Build history of the part. All positions in model axes, mm. A direction names the side the tool comes from. Coordinates: 2 decimals unless noted, no trailing zeros. Loops run counter-clockwise (first coordinate to the right, second up) from the corner with the lowest first, then second, coordinate; pieces in that order, holes last.
(1) Tool access for faces 1 (the face through (-83.577, 56.38, -1.565)), 2 (the face through (-75, 46, -91.148)), 3 (the face through (-78.03, 49.35, -92.71)), 4 (the face through (-66.658, 34.949, -1.565)), 5 (the face through (-75, 46, -3.175)): list every direction of +Z, -Z, +X, -X, +Y, -Y with a clear straight run to the whole face (end or side of a thin tool).
(2) Wall check: L1, parallel to Z at x = -86.5, y = 60 (3 decimals); L2, parallel to X at y = 50, z = -16; L3, parallel to X at y = 59.5, z = -41. Give the ranges that are in metal, low to high.
(3) Slice it at A-A (x = -67). Give the cut face in (y, z) (3 decimals), and give its area (3 significant figures).
(4) Slice it at B-B (z = -26.5). Give the cut face in (x, y), and give its area (3 significant figures).
(5) Slice it at C-C (y = 27). Give the cut face in (x, z) (3 decimals).
(6) Flat gauge pins, fed straight in: P1, Ø11.5, axis at x = -61.5, y = 28.5, coming from the -Z side; P2, Ø2, axis at y = 53, z = -75.5, coming from the +X side; P3, Ø8, axis at x = -72, y = 34, coming from the +Z side; P4, Ø3, axis at x = -63.5, y = 30, coming from the +Z side (3 decimals). Where does each tip first touch, or does it go through?
from build123d import *

# Parameters (mm, degrees)
BOSS_EXTRUDE1_DEPTH = 94.322511
SKETCH2_W           = 3.175
SKETCH2_H           = 12.7
SKETCH2_H_2         = 9.525
CUT_EXTRUDE1_DEPTH  = 146.131101822


with BuildPart() as part:
    # Sketch1 → Boss-Extrude1 (new body)
    with BuildSketch(Plane.XY):
        Polygon((-57.559752251, 25.95051887), (-90.217961646, 67.317584104), (-92.709964426, 65.350213488), (-60.051755031, 23.983148254), align=None)
    extrude(amount=-BOSS_EXTRUDE1_DEPTH)

    # Sketch2 → Cut-Extrude1 (cut, through all)
    with BuildSketch(Plane(origin=(-22.838178642, -18.030141034, 0), x_dir=(0, 0, -1), z_dir=(0.7848827655333936, 0.6196442885790622, 0))):
        with Locations((92.735011379, 102.389456242)):
            Rectangle(SKETCH2_W, SKETCH2_H)
        with Locations((92.735011379, 82.323686752)):
            Rectangle(SKETCH2_W, SKETCH2_H_2)
        with Locations((92.735011379, 62.384686752)):
            Rectangle(SKETCH2_W, SKETCH2_H)
        with Locations((1.5875, 102.389456242)):
            Rectangle(SKETCH2_W, SKETCH2_H)
        with Locations((1.5875, 82.323686752)):
            Rectangle(SKETCH2_W, SKETCH2_H_2)
        with Locations((1.5875, 62.384686752)):
            Rectangle(SKETCH2_W, SKETCH2_H)
    extrude(amount=-CUT_EXTRUDE1_DEPTH, mode=Mode.SUBTRACT)


solid = part.part
Response values:
1. face 1: +Z, -X, +Y
1. face 2: -Z
1. face 3: -Z, +X, -Y
1. face 4: +Z, +X, -Y
1. face 5: +Z
2. L1: z = -91.148 to -3.175
2. L2: x = -80.59 to -76.55
2. L3: x = -88.09 to -84.05
3. outline: (32.784, -91.148) - (34.678, -91.148) - (34.678, -94.323) - (37.908, -94.323) - (37.908, 0) - (34.678, 0) - (34.678, -3.175) - (32.784, -3.175) - close
3. area: 471 mm2
4. outline: (-92.71, 65.35) - (-60.05, 23.98) - (-57.56, 25.95) - (-90.22, 67.32) - close
4. area: 167 mm2
5. outline: (-62.433, -91.148) - (-58.388, -91.148) - (-58.388, -3.175) - (-62.433, -3.175) - close
6. P1: stops at z = -91.15
6. P2: stops at x = -78.13
6. P3: stops at z = 0
6. P4: stops at z = -3.175
